```python
from build123d import *

# Parameters (mm, degrees)
F0_W     = 86.9941338897
F0_H     = 125.2852901816
F1_DEPTH = 25.4
F2_DEPTH = 25.4
F4_D     = 6.35
F5_DEPTH = 25.4


with BuildPart() as f1:
    # F0 (on Top) → F1 (new body)
    with BuildSketch(Plane.XY):
        with Locations((5.0123818219, 15.9891955554)):
            Rectangle(F0_W, F0_H)
    extrude(amount=F1_DEPTH)

    # F2 (add): a face of the model
    f2_faces = [f1.faces().sort_by_distance(p)[0] for p in [
        (5.0123818219, -46.6534495354, 12.7),
    ]]
    extrude(f2_faces, amount=F2_DEPTH)

    # F4 (through all)
    with Locations(Plane.XY.offset(25.4)):
        with Locations((0, 0)):
            Hole(F4_D / 2)

    # F5 (add): a face of the model
    f5_faces = [f1.faces().sort_by_distance(p)[0] for p in [
        (5.0245204925, 3.2971611221, 25.4),
    ]]
    extrude(f5_faces, amount=F5_DEPTH)


solid = f1.part
```
Part model, mm, in its own coordinate system. Round coordinates to 2 decimals unless told otherwise and drop trailing zeros. Loops run counter-clockwise (first coordinate to the right, second up) from the corner with the lowest first, then second, coordinate; pieces in that order, holes last. Notation, with made-up numbers: (53, -4.75) -> (74, -4.75) arc R28 ccw to (74, 19.25) -> close; hole circle Ø1 at (1.5, 17.5). An arc over 180 degrees is marked (long way). Use CSV: the item, a comma, the result in double quotes. Start each with the question number.
1) Pull direction X, two halves, no side cores. Call faces 1 (the flat face through (48.509, 2, 25)), 2 (the flat face through (4, 4, 0)), 3 (the cylindrical face through (0.69, -3.1, 25.04)): +X half, -X half, draft (parallel to the pull), parting line (faces both ways), or undercut.
2) Cut at B-B, the plane y = 0. Write the cut outline in (x, z) (3 decimals), plus the area to 3 significant figures.
3) Cut at A-A, the plane x = 0. Write the cut outline in (y, z) (3 decimals).
4) Wall check: L1, parallel to Y at x = 0, z = 30 (3 decimals). Give the ranges that are in metal, low to high. Write a range as [from, to].
Determined:
1,face 1,"+X half"
1,face 2,"draft"
1,face 3,"undercut"
2,outline,"(-38.485, 0) -> (-3.175, 0) -> (-3.175, 50.8) -> (-38.485, 50.8) -> close; (3.175, 0) -> (48.509, 0) -> (48.509, 50.8) -> (3.175, 50.8) -> close"
2,area,"4,100 mm2"
3,outline,"(-72.053, 0) -> (-3.175, 0) -> (-3.175, 50.8) -> (-72.053, 50.8) -> close; (3.175, 0) -> (78.632, 0) -> (78.632, 50.8) -> (3.175, 50.8) -> close"
4,L1,"y = [-72.053, -3.175], [3.175, 78.632]"
